Answer from the drawing. Dimensions are ordinates in mm from the lowest x, y and z of the part. Coordinates: 2 decimals unless noted, no trailing zeros. Write each loop counter-clockwise with the first axis right and the second up, starting at its lowest first coordinate (ties: lowest second). Pieces come first, ordered by that corner, then holes. Notation, with made-up numbers: (-12.5, 87) -> (46.5, 87) arc R33 cw to (46.5, 124) -> close; hole circle Ø10 at (39.25, 40). An arc over 180 degrees is marked (long way). One line per item, written item: value. Start each with the question number.
1. Consider line 1 along Z through (x, y) = (4.5, 6.25) (1 decimal); line 2 along Y through (x, z) = (5, 20.25) (1 decimal). Determine where each line is inside the solid, lowest interval first.
2. Find section A-A, the plane y = 4.5. State how many separate pieces and enclosed holes the cut face has, and give its area (3 significant figures).
3. Given P1, Ø2.5, axis at x = 4.76, z = 19.05, coming from the -Y side (1 decimal), flat-ended and moving along its own axis, determine where the tip first touches the part or whether it passes through.
4. For a pull along Z with two mould halves and no side action, classify the marked faces 1, 2, 3 and 4 as pulls with the +Z half, pulls with the -Z half, needs draft (parallel to the pull), parting line crosses it, or undercut.
5. Find section D-D, the plane z = 7.5. Write down the section's boundary in (x, y) (1 decimal), and give its area (3 significant figures).
6. Find section C-C, the plane x = 4. Write down the section's boundary in (y, z) (1 decimal).
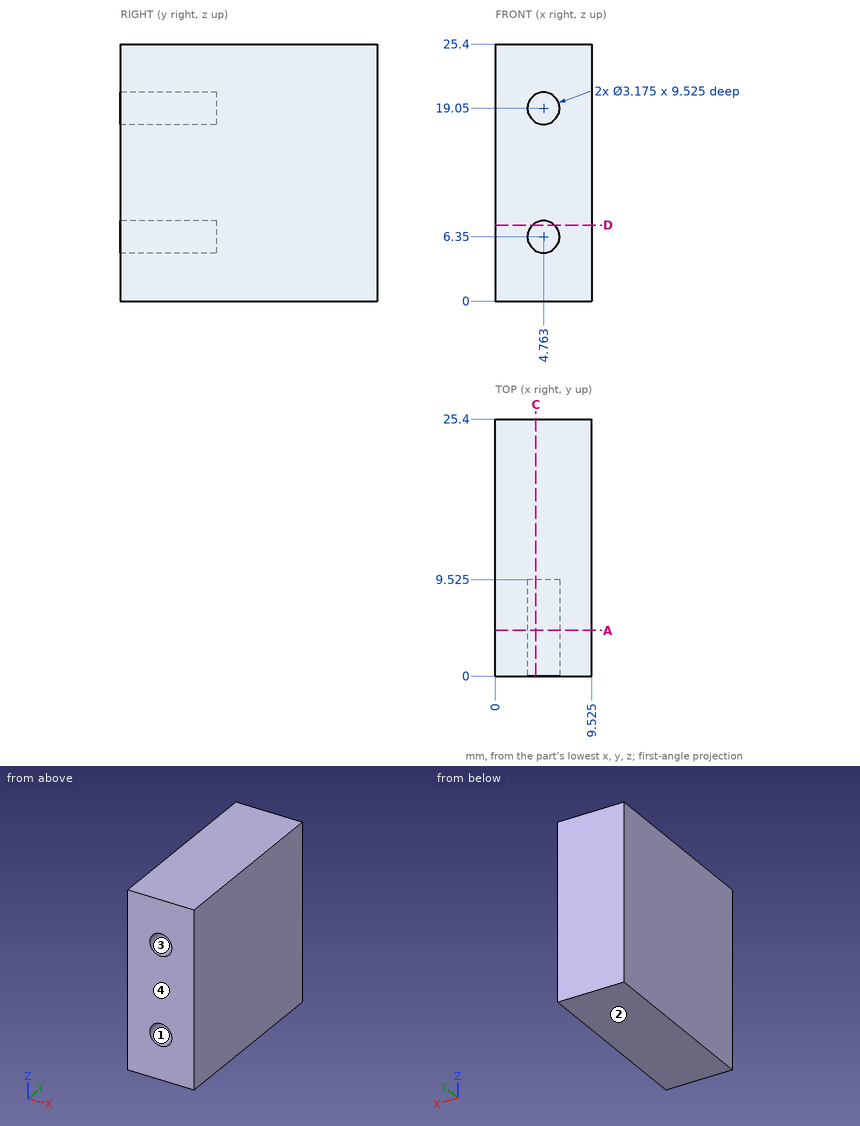
Answer block:
1. line 1: z = 0 to 4.8, 7.9 to 17.5, 20.6 to 25.4
1. line 2: y = 9.5 to 25.4
2. separate pieces: 1
2. enclosed holes: 2
2. area: 226 mm2
3. P1: stops at y = 9.5
4. face 1: undercut
4. face 2: pulls with the -Z half
4. face 3: undercut
4. face 4: needs draft
5. outline: (0, 0) -> (3.7, 0) -> (3.7, 9.5) -> (5.9, 9.5) -> (5.9, 0) -> (9.5, 0) -> (9.5, 25.4) -> (0, 25.4) -> close
5. area: 221 mm2
6. outline: (0, 0) -> (25.4, 0) -> (25.4, 25.4) -> (0, 25.4) -> (0, 20.4) -> (9.5, 20.4) -> (9.5, 17.7) -> (0, 17.7) -> (0, 7.7) -> (9.5, 7.7) -> (9.5, 5) -> (0, 5) -> close
